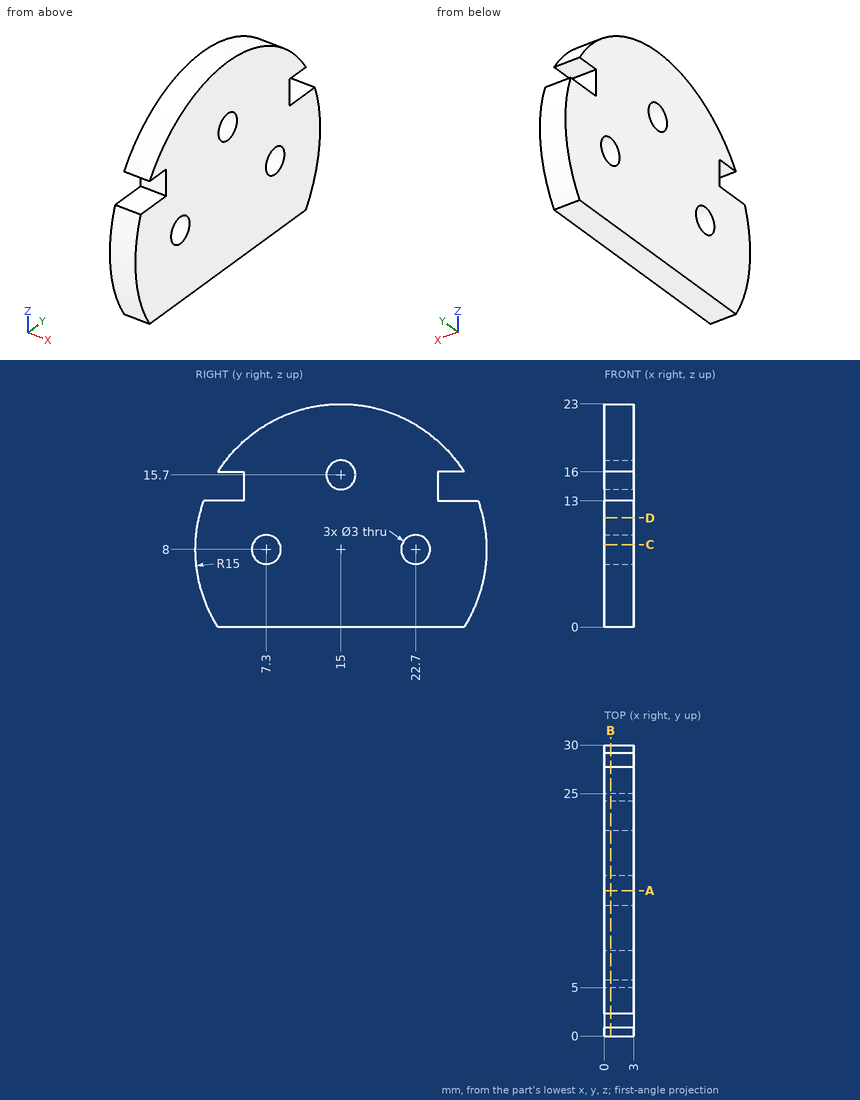
Here's the drawing with two shaded views (mm, measured from the low corner). I have some questions. Round coordinates to 2 decimals unless told otherwise and drop trailing zeros. Order: outer loops, then holes, each group sorted by start corner. A loop starts at its lowest first (then second) coordinate and runs counter-clockwise, first axis right, second up. Notation, with made-up numbers: M -3.75,-15.75 L 11.25,-15.75 A12 ccw 11.25,2.25 Z; hole C -31,67.25 d4. An arc over 180 degrees is marked long. Use CSV: the item, a comma, the result in double quotes.
1) I want a section at C-C (z = 8.5). List the corners of the cut face in (x, y) for me.
Taken from the geometry:
outline,"M 0,0.01 L 3,0.01 L 3,5.89 L 0,5.89 Z; M 0,8.71 L 3,8.71 L 3,21.29 L 0,21.29 Z; M 0,24.11 L 3,24.11 L 3,29.99 L 0,29.99 Z"
2) I want a section at B-B (x = 0.65). List the corners of the cut face in (y, z) for me, then the cut area to 3 significant figures.
Taken from the geometry:
outline,"M 0.86,13 A15 ccw 2.31,0 L 27.69,0 A15 ccw 29.14,13 L 25,13 L 25,16 L 27.69,16 A15 ccw 2.31,16 L 5,16 L 5,13 Z; hole C 7.3,8 d3; hole C 15,15.7 d3; hole C 22.7,8 d3"
area,"539 mm^2"
3) I want a section at D-D (z = 11.25). List the corners of the cut face in (x, y) for me, then the cut area to 3 significant figures.
Taken from the geometry:
outline,"M 0,0.36 L 3,0.36 L 3,29.64 L 0,29.64 Z"
area,"87.9 mm^2"
4) I'm going to push flat-ended pins straight in: P1, Ø0.9, axis at x = 1.5, z = 14.5, coming from the +Y side; P2, Ø1, axis at x = 1, y = 14, coming from the +Z side; P3, Ø0.9, axis at x = 1, y = 27, coming from the +Z side. Where does each tip first touch, or does it pass through?
Taken from the geometry:
P1,"y = 25"
P2,"z = 22.99"
P3,"z = 17.57"
5) I need wall thicknesses on line 1 along Y through (x, z) = (1.15, 8); line 2 along Z through (x, y) = (1.45, 15); line 3 along Z through (x, y) = (1.3, 22.7). Which ranges of each line are inside material? Lowest first, please. Write a range as [from, to].
Taken from the geometry:
line 1,"[0, 5.8], [8.8, 21.2], [24.2, 30]"
line 2,"[0, 14.2], [17.2, 23]"
line 3,"[0, 6.5], [9.5, 20.87]"
6) I want a section at A-A (y = 15). List the corners of the cut face in (x, z) for me, then the cut area to 3 significant figures.
Taken from the geometry:
outline,"M 0,0 L 3,0 L 3,14.2 L 0,14.2 Z; M 0,17.2 L 3,17.2 L 3,23 L 0,23 Z"
area,"60.0 mm^2"
